Autodesk Inventor part; units mm, degrees
ref_plane "YZ Plane" through (0, 0, 0) normal (1, 0, 0) x (0, 1, 0)
ref_plane "XZ Plane" through (0, 0, 0) normal (0, 1, 0) x (-1, 0, 0)
ref_plane "XY Plane" through (0, 0, 0) normal (0, 0, 1) x (1, 0, 0)
sketch "Sketch1" plane through (0, 0, 0) normal (0, 0, 1) x (1, 0, 0)
  line L0 (0, 0) -> (15.875, 0)
  line L1 (15.875, 0) -> (15.875, 0.7937)
  line L2 (15.875, 0.7937) -> (0.7938, 0.7937)
  line L3 (0.7938, 0.7937) -> (0.7937, 15.875)
  line L4 (0.7937, 15.875) -> (0, 15.875)
  line L5 (0, 15.875) -> (0, 0)
  dimension "d0" = 15.875
  dimension "d1" = 0.7937
  dimension "d2" = 0.7937
extrude "Extrusion1" add sketch "Sketch1" along normal blind 474.6752
sketch "Sketch2" plane through (0.7937, 0.7937, 0) normal (1, 0, 0) x (0, 0, -1)
  line L0 (0, 0) -> (0, 15.0812)
  line L1 (-474.6752, 0) -> (-474.6752, 15.0812)
  line L2 (-474.6752, 7.5406) -> (0, 7.5406) construction
  circle A0 centre (-455.6252, 112.4267) radius 2.2479 construction
  circle A1 centre (-82.55, 112.4267) radius 2.2479 construction
  circle A2 centre (-63.5127, 112.4267) radius 2.2479 construction
  circle A3 centre (-19.0627, 112.4267) radius 2.2479 construction
  circle A4 centre (-6.35, 112.4267) radius 2.2479 construction
  circle A5 centre (-246.0752, 112.4267) radius 2.2479 construction
  circle A6 centre (-347.6752, 112.4267) radius 2.2479 construction
  line L3 (0, 104.8861) -> (0, 119.9674) construction
  line L4 (0, 119.9674) -> (-474.6752, 119.9674) construction
  line L5 (-474.6752, 104.8861) -> (-474.6752, 119.9674) construction
  line L6 (0, 104.8861) -> (-474.6752, 104.8861) construction
  circle A7 centre (-455.6252, 7.5406) radius 2.2479
  circle A8 centre (-347.6752, 7.5406) radius 2.2479
  circle A9 centre (-246.0752, 7.5406) radius 2.2479
  circle A10 centre (-82.55, 7.5406) radius 2.2479
  circle A11 centre (-6.35, 7.5406) radius 2.2479
  line L7 (-455.6252, 112.4267) -> (-455.6252, 7.5406) construction
  line L8 (-347.6752, 7.5406) -> (-347.6752, 112.4267) construction
  line L9 (-246.0752, 112.4267) -> (-246.0752, 7.5406) construction
  line L10 (-82.55, 112.4267) -> (-82.55, 7.5406) construction
  line L11 (-6.35, 7.5406) -> (-6.35, 112.4267) construction
  circle A12 centre (-330.2127, 8.7312) radius 1.905
  circle A13 centre (-369.6843, 112.9728) radius 1.905
  point P0 (0, -0.7937)
extrude "Extrusion2" cut sketch "Sketch2" against normal through all contours A7 | A8 | A9 | A10 | A11 | A12
properties part number "Electrical Board 1 Bracing L Channel Part 2" material "Aluminum 6061"
Verification items for the finished model (mm, model axes). A direction names the side the tool comes from. Round coordinates to 2 decimals unless told otherwise and drop trailing zeros. Write each loop counter-clockwise with the first axis right and the second up, starting at its lowest first coordinate (ties: lowest second). Pieces come first, ordered by that corner, then holes.
1. Gauge pin test, flat ends, axial feed: P1, Ø7, axis at y = 8.33, z = 82.55, coming from the -X side; P2, Ø3.5, axis at y = 8.33, z = 455.63, coming from the +X side; P3, Ø4.5, axis at x = 7, z = 206, coming from the +Y side; P4, Ø5, axis at y = 9.52, z = 330.21, coming from the +X side. Record the tip position at first contact, or that the pin passes through.
2. Section check B-B on x = 9.25. Enter the section's corners in (y, z).
3. Access from +Z, -Z, +X, -X, +Y, -Y to the whole of each face (thin tool, end or side, straight path). Record for faces 1 (the flat face through (0, 8, 234)), 2 (the flat face through (8, 0.794, 234)).
4. Section check A-A on z = 292. Enter the section's corners in (x, y) (3 decimals).
5. Scan lines: L1, parallel to Y at x = 0.65, z = 82.55 (3 decimals); L2, parallel to Y at x = 11.5, z = 269. Record each from-to range of solid material in increasing order.
Answer:
1. P1: stops at x = 0
1. P2: passes through
1. P3: stops at y = 0.79
1. P4: stops at x = 0.79
2. outline: (0, 0) - (0.79, 0) - (0.79, 474.68) - (0, 474.68) - close
3. face 1: +Z, -Z, -X, +Y, -Y
3. face 2: +Z, -Z, +X, +Y
4. outline: (0, 0) - (15.875, 0) - (15.875, 0.794) - (0.794, 0.794) - (0.794, 15.875) - (0, 15.875) - close
5. L1: y = 0 to 6.086, 10.582 to 15.875
5. L2: y = 0 to 0.79
